Can you work these out from the model? Positions are in its coordinate system, mm. Face numbers are marked on the shaded views. A direction names the side the tool comes from. Coordinates: 2 decimals unless noted, no trailing zeros. Order: outer loops, then holes, each group sorted by start corner. A loop starts at its lowest first (then second) coordinate and runs counter-clockwise, first axis right, second up.
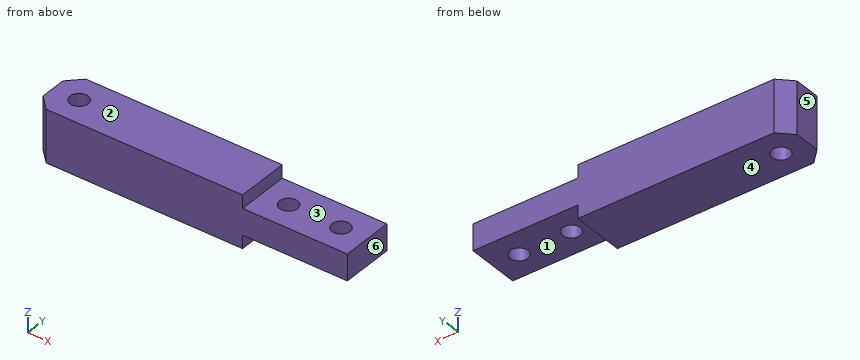
```python
from build123d import *

# Parameters (mm, degrees)
BOSS_EXTRUDE1_DEPTH     = 6.35
CUT_EXTRUDE1_DEPTH      = 78.51162816
CUT_EXTRUDE1_DEPTH_BACK = 78.51162816
SKETCH2_R               = 2.1828125
CHAMFER1_SIZE           = 3.175


with BuildPart() as part:
    # Sketch1 → Boss-Extrude1 (new, symmetric)
    with BuildSketch(Plane(origin=(0, 0, 0), x_dir=(1, 0, 0), z_dir=(0, 1, 0))):
        Polygon((0, 0), (50.8, 0), (50.8, 3.175), (76.2, 3.175), (76.2, 9.525), (50.8, 9.525), (50.8, 12.7), (0, 12.7), align=None)
    extrude(amount=BOSS_EXTRUDE1_DEPTH, both=True)

    # Sketch2 → Cut-Extrude1 (cut, two sides: drawn at the far end of the back side and taken through both)
    with BuildSketch(Plane.XY.offset(-CUT_EXTRUDE1_DEPTH_BACK)):
        with Locations((6.35, 0)):
            Circle(SKETCH2_R)
        with Locations((57.15, 0)):
            Circle(SKETCH2_R)
        with Locations((69.85, 0)):
            Circle(SKETCH2_R)
    extrude(amount=CUT_EXTRUDE1_DEPTH + CUT_EXTRUDE1_DEPTH_BACK, mode=Mode.SUBTRACT)

    # Chamfer1
    chamfer1_edges = [part.edges().sort_by_distance(p)[0] for p in [
        (0, -6.35, -6.35),
        (0, 6.35, -6.35),
    ]]
    chamfer(chamfer1_edges, length=CHAMFER1_SIZE)


solid = part.part
```
1. Imagine slicing it at D-D on z = -7.25. Please give me the cut outline in (x, y) (3 decimals), then the cut area to 3 significant figures.
Completed:
outline: (0, -3.175) - (3.175, -6.35) - (76.2, -6.35) - (76.2, 6.35) - (3.175, 6.35) - (0, 3.175) - close; hole circle Ø4.366 at (6.35, 0); hole circle Ø4.366 at (57.15, 0); hole circle Ø4.366 at (69.85, 0)
area: 913 mm2
2. Imagine slicing it at C-C on z = -10.75. Please give me the cut outline in (x, y) (3 decimals).
Completed:
outline: (0, -3.175) - (3.175, -6.35) - (50.8, -6.35) - (50.8, 6.35) - (3.175, 6.35) - (0, 3.175) - close; hole circle Ø4.366 at (6.35, 0)
3. Imagine slicing it at B-B on x = 6.35. Please give me the cut outline in (y, z).
Completed:
outline: (-6.35, -12.7) - (-2.18, -12.7) - (-2.18, 0) - (-6.35, 0) - close; (2.18, -12.7) - (6.35, -12.7) - (6.35, 0) - (2.18, 0) - close
4. Imagine slicing it at A-A on y = 0. Please give me the cut outline in (x, z) (3 decimals).
Completed:
outline: (0, -12.7) - (4.167, -12.7) - (4.167, 0) - (0, 0) - close; (8.533, -12.7) - (50.8, -12.7) - (50.8, -9.525) - (54.967, -9.525) - (54.967, -3.175) - (50.8, -3.175) - (50.8, 0) - (8.533, 0) - close; (59.333, -9.525) - (67.667, -9.525) - (67.667, -3.175) - (59.333, -3.175) - close; (72.033, -9.525) - (76.2, -9.525) - (76.2, -3.175) - (72.033, -3.175) - close
5. Thinking about a two-plate mould opening in X: for the marked faces 4, 5 and 6, which applies, pulls with the +X half, pulls with the -X half, needs draft (parallel to the pull), parting line crosses it, or undercut?
Completed:
face 4: needs draft
face 5: pulls with the -X half
face 6: pulls with the +X half
6. I'm going to push flat-ended pins straight in: pin 1 (4 mm diameter, centred on x = 63.5, y = 1, fed in from -Z) (3 decimals); pin 2 (4 mm diameter, centred on x = 68, y = 1.5, fed in from +Z) (3 decimals). Where does each tip first touch, or does it pass through?
Completed:
pin 1: stops at z = -9.525
pin 2: stops at z = -3.175
7. On a 3-axis mill with a long thin cutter (end or side, diameter ignored), from which of +Z, -Z, +X, -X, +Y, -Y can I reach the whole of each face in a straight line? I mean the marked faces 1, 2 and 3. Say none if no direction works.
Completed:
face 1: -Z, +X, +Y, -Y
face 2: +Z, +X, -X, +Y, -Y
face 3: +Z, +X, +Y, -Y
8. Please list where these lines run through material, in increasing order: probe 1 along X at (y, z) = (0, -3.5); probe 2 along X at (y, z) = (0, -2.5); probe 3 along Y at (x, z) = (69.85, -6.75).
Completed:
probe 1: x = 0 to 4.17, 8.53 to 54.97, 59.33 to 67.67, 72.03 to 76.2
probe 2: x = 0 to 4.17, 8.53 to 50.8
probe 3: y = -6.35 to -2.18, 2.18 to 6.35
